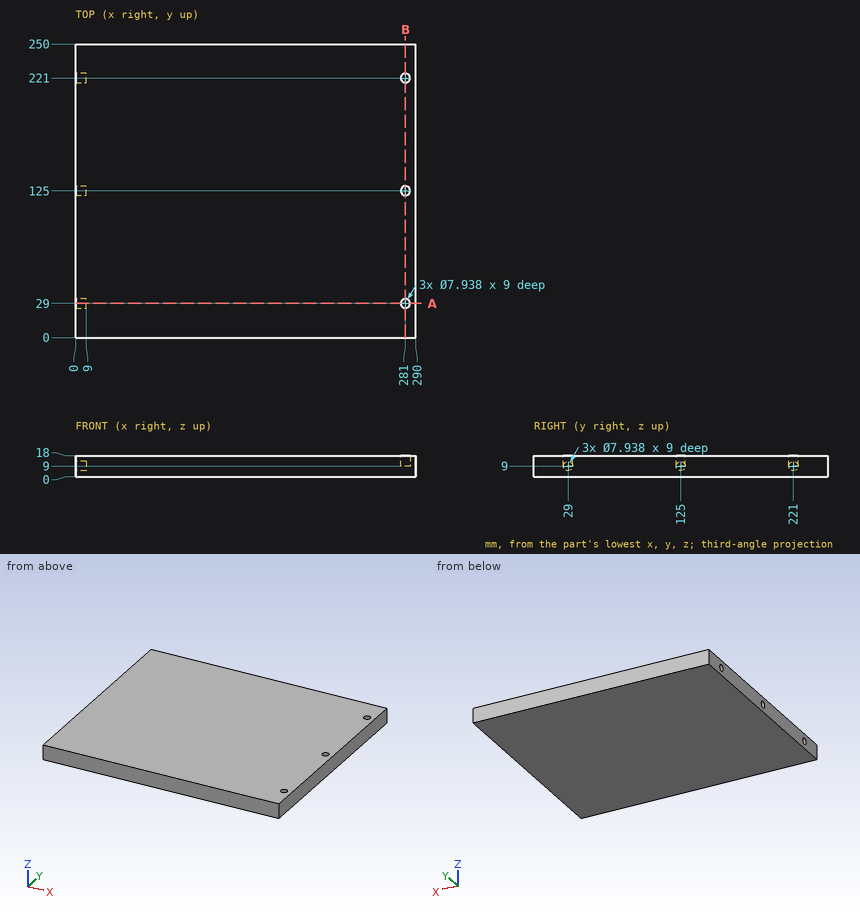
Part print with two shaded views. Sizes in mm from the minimum x, y, z corner. Give positions to 0.01 mm unless a question says otherwise; leave off trailing zeros. Order: outer loops, then holes, each group sorted by start corner. A loop starts at its lowest first (then second) coordinate and runs counter-clockwise, first axis right, second up.
(1) Saw through at B-B, the plane x = 281. Give the cut face in (y, z), then the cut area to 3 significant figures.
(2) Saw through at A-A, the plane y = 29. Give the cut face in (x, z), then the cut area to 3 significant figures.
(3) Flat gauge pins, fed straight in: pin 1 (2.5 mm diameter, centred on x = 279.5, y = 222.5, fed in from +Z); pin 2 (6.5 mm diameter, centred on y = 125, z = 9, fed in from -X). Where does each tip first touch, or does it go through?
(4) Drill centre lines: L1, parallel to Y at x = 281, z = 16; L2, parallel to Z at x = 4, y = 29; L3, parallel to X at y = 26, z = 16 (1 decimal). Where is each one in solid material? Low to high.
Results found:
1. outline: (0, 0) - (250, 0) - (250, 18) - (224.97, 18) - (224.97, 9) - (217.03, 9) - (217.03, 18) - (128.97, 18) - (128.97, 9) - (121.03, 9) - (121.03, 18) - (32.97, 18) - (32.97, 9) - (25.03, 9) - (25.03, 18) - (0, 18) - close
1. area: 4,290 mm2
2. outline: (0, 0) - (290, 0) - (290, 18) - (284.97, 18) - (284.97, 9) - (277.03, 9) - (277.03, 18) - (0, 18) - (0, 12.97) - (9, 12.97) - (9, 5.03) - (0, 5.03) - close
2. area: 5,080 mm2
3. pin 1: stops at z = 9
3. pin 2: stops at x = 9
4. L1: y = 0 to 25.03, 32.97 to 121.03, 128.97 to 217.03, 224.97 to 250
4. L2: z = 0 to 5.03, 12.97 to 18
4. L3: x = 0 to 278.4, 283.6 to 290
